Could you check a few things on this model? Use its own coordinates, in mm. A direction names the side the tool comes from. Give positions to 0.01 mm unless a question says otherwise; leave off trailing zeros. Loops run counter-clockwise (first coordinate to the right, second up) from the corner with the lowest first, then second, coordinate; pieces in that order, holes last. Notation, with made-up numbers: M -31,-23.5 L -16,-23.5 A15 ccw -16,-9.5 Z; hole C 43,11 d8. An arc over 180 degrees is marked long. Answer in a Markdown table with one row per item. Add a question column.
```python
from build123d import *

# Parameters (mm, degrees)
ESQUISSE1_W                  = 60
ESQUISSE1_H                  = 60
BOSS_EXTRU_1_DEPTH           = 3
ESQUISSE2_W                  = 40
ESQUISSE2_H                  = 5.064093089
BOSS_EXTRU_2_DEPTH           = 60
ESQUISSE3_R                  = 2.1
ESQUISSE3_W                  = 21
ESQUISSE3_H                  = 42.4
ENL_V_MAT_EXTRU_1_DEPTH      = 61
ESQUISSE4_W                  = 31.43634342
ESQUISSE4_H                  = 7.471813822
BOSS_EXTRU_3_DEPTH           = 49
ENL_V_MAT_EXTRU_2_DEPTH      = 49
ENL_V_MAT_EXTRU_2_DEPTH_BACK = 49
ESQUISSE5_R                  = 2.1
ENL_V_MAT_EXTRU_3_DEPTH      = 5
ENL_V_MAT_EXTRU_3_DEPTH_BACK = 12
ENL_V_MAT_EXTRU_7_DEPTH      = 5.686588472
BOSS_EXTRU_4_DEPTH           = 5
ESQUISSE13_R                 = 1.5
ENL_V_MAT_EXTRU_8_DEPTH      = 5
ENL_V_MAT_EXTRU_9_DEPTH      = 10
CHANFREIN1_SIZE              = 3
CHANFREIN2_SIZE              = 3
ESQUISSE15_R                 = 40.585379392
BOSS_EXTRU_5_DEPTH           = 3
ESQUISSE16_R                 = 4
BOSS_EXTRU_6_DEPTH           = 5.5
ESQUISSE17_R                 = 34
ESQUISSE17_R_2               = 31
BOSS_EXTRU_7_DEPTH           = 1.5


with BuildPart() as part:
    # Esquisse1 → Boss.-Extru.1 (new body)
    with BuildSketch(Plane(origin=(0, 0, 0), x_dir=(1, 0, 0), z_dir=(0, 1, 0))):
        Rectangle(ESQUISSE1_W, ESQUISSE1_H)
    extrude(amount=BOSS_EXTRU_1_DEPTH)

    # Esquisse2 → Boss.-Extru.2 (add)
    with BuildSketch(Plane(origin=(0, 3, 0), x_dir=(1, 0, 0), z_dir=(0, 1, 0))):
        with Locations((0, -27.467953456)):
            Rectangle(ESQUISSE2_W, ESQUISSE2_H)
        with Locations((0, 27.467953456)):
            Rectangle(ESQUISSE2_W, ESQUISSE2_H)
    extrude(amount=BOSS_EXTRU_2_DEPTH)

    # Esquisse3 → Enlèv. mat.-Extru.1 (cut)
    with BuildSketch(Plane.XY.offset(30)):
        with Locations((-5, 57.819250322)):
            Circle(ESQUISSE3_R)
        with Locations((5, 57.819250322)):
            Circle(ESQUISSE3_R)
        with Locations((-5, 7.419250322)):
            Circle(ESQUISSE3_R)
        with Locations((5, 7.419250322)):
            Circle(ESQUISSE3_R)
        with Locations((0, 32.619250322)):
            Rectangle(ESQUISSE3_W, ESQUISSE3_H)
    extrude(amount=-ENL_V_MAT_EXTRU_1_DEPTH, mode=Mode.SUBTRACT)

    # Esquisse4 → Boss.-Extru.3 (add)
    with BuildSketch(Plane(origin=(0, 3, 0), x_dir=(1, 0, 0), z_dir=(0, 1, 0))):
        with Locations((0, 8.9)):
            Rectangle(ESQUISSE4_W, ESQUISSE4_H)
    extrude(amount=BOSS_EXTRU_3_DEPTH)

    # Esquisse5 → Enlèv. mat.-Extru.2 (cut, two sides: drawn at the far end of the back side and taken through both)
    with BuildSketch(Plane.XY.offset(-5.164093089).offset(-ENL_V_MAT_EXTRU_2_DEPTH_BACK)):
        with Locations(Location((0, 41.884866589, 0), (0, 0, 180))):
            Circle(ESQUISSE5_R)
    extrude(amount=ENL_V_MAT_EXTRU_2_DEPTH + ENL_V_MAT_EXTRU_2_DEPTH_BACK, mode=Mode.SUBTRACT)

    # Esquisse6 → Enlèv. mat.-Extru.3 (cut, two sides: drawn at the far end of the back side and taken through both)
    with BuildSketch(Plane.XY.offset(-5.164093089).offset(-ENL_V_MAT_EXTRU_3_DEPTH_BACK)):
        Polygon((3.765814794, 52), (-3.765814794, 52), (-8.396406616, 48.113602092), (-13.009515703, 41.697186725), (-16.070942643, 28.570794505), (-19.383993714, 28.570794505), (-19.383993714, 55.569676943), (19.383993714, 55.569676943), (19.383993714, 28.570794505), (16.070942643, 28.570794505), (13.009515703, 41.697186725), (8.396406616, 48.113602092), align=None)
    extrude(amount=ENL_V_MAT_EXTRU_3_DEPTH + ENL_V_MAT_EXTRU_3_DEPTH_BACK, mode=Mode.SUBTRACT)

    # Esquisse11 → Enlèv. mat.-Extru.7 (cut)
    with BuildSketch(Plane.XY.offset(30)):
        Polygon((-3.554651837, 53.819250322), (0, 57.156758738), (3.554651837, 53.819250322), align=None)
        Polygon((3.554651837, 11.419250322), (0.008232601, 8.05699671), (-3.554651837, 11.419250322), align=None)
    enl_v_mat_extru_7 = extrude(amount=-ENL_V_MAT_EXTRU_7_DEPTH, mode=Mode.SUBTRACT)

    # Symétrie1: Enlèv. mat.-Extru.7 across plane
    add(enl_v_mat_extru_7.mirror(Plane.XY), mode=Mode.SUBTRACT)

    # Esquisse12 → Boss.-Extru.4 (add)
    with BuildSketch(Plane(origin=(0, 0, -30), x_dir=(-1, 0, 0), z_dir=(0, 0, -1))):
        Polygon((-16.041577075, 53.722563772), (-27.510987985, 61.809968901), (-27.510987985, 29.990434482), (-16.041577075, 21.903029354), align=None)
    extrude(amount=-BOSS_EXTRU_4_DEPTH)

    # Esquisse13 → Enlèv. mat.-Extru.8 (cut)
    with BuildSketch(Plane(origin=(0, 0, -30), x_dir=(-1, 0, 0), z_dir=(0, 0, -1))):
        with Locations((-23.733778696, 54.232255727)):
            Circle(ESQUISSE13_R)
    extrude(amount=-ENL_V_MAT_EXTRU_8_DEPTH, mode=Mode.SUBTRACT)

    # Esquisse14 → Enlèv. mat.-Extru.9 (cut)
    with BuildSketch(Plane(origin=(0, 0, -30), x_dir=(-1, 0, 0), z_dir=(0, 0, -1))):
        with BuildLine():
            Line((-21.71817898, 57.725295885), (-22.313097289, 61.571545457))
            Line((-22.313097289, 61.571545457), (-29.123823422, 63.566297114))
            Line((-29.123823422, 63.566297114), (-31.434035617, 54.282245365))
            Line((-31.434035617, 54.282245365), (-31.802093045, 39.80867485))
            Line((-31.802093045, 39.80867485), (-27.510987985, 39.80867485))
            add(Edge.make_bspline(
                [(-27.510987985, 39.80867485), (-27.476511879, 42.426218442), (-27.330002572, 45.177230576), (-27.18875986, 50.317216066), (-27.834123365, 55.293883989), (-23.939343069, 59.432145797), (-21.71817898, 57.725295885)],
                knots=[0, 0, 0, 0, 0.330124206, 0.401515798, 0.713915923, 1, 1, 1, 1], degree=3))
        make_face()
    extrude(amount=-ENL_V_MAT_EXTRU_9_DEPTH, mode=Mode.SUBTRACT)

    # Chanfrein1
    chanfrein1_edges = [part.edges().sort_by_distance(p)[0] for p in [
        (-20, 63, 27.467953456),
        (20, 63, 27.467953456),
        (20, 63, -27.467953456),
        (-20, 63, -27.467953456),
    ]]
    chamfer(chanfrein1_edges, length=CHANFREIN1_SIZE)

    # Chanfrein2
    chanfrein2_edges = [part.edges().sort_by_distance(p)[0] for p in [
        (15.71817171, 3, -8.9),
        (0, 3, -12.635906911),
        (-15.71817171, 3, -8.9),
        (0, 3, -5.164093089),
    ]]
    chamfer(chanfrein2_edges, length=CHANFREIN2_SIZE)

    # Esquisse15 → Boss.-Extru.5 (add)
    with BuildSketch(Plane.XZ):
        Circle(ESQUISSE15_R)
    extrude(amount=-BOSS_EXTRU_5_DEPTH)

    # Esquisse16 → Boss.-Extru.6 (add)
    with BuildSketch(Plane.XZ):
        with Locations(Location((0, 0, 0), (0, 0, 90))):
            Circle(ESQUISSE16_R)
        with BuildLine():
            Line((1.5, -2), (-1.5, -2))
            add(Edge.make_bspline(
                [(-1.5, 2), (-1.958697555, 1.657983746), (-2.533324792, 0.788068376), (-2.517224478, -0.822180507), (-1.942930835, -1.670082257), (-1.5, -2)],
                knots=[0, 0, 0, 0, 0.368917338, 0.642208585, 1, 1, 1, 1], degree=3))
            Line((-1.5, 2), (1.5, 2))
            add(Edge.make_bspline(
                [(1.5, 2), (1.95810566, 1.657096874), (2.561237256, 0.750226685), (2.498088101, -0.878428585), (1.905080516, -1.696028501), (1.5, -2)],
                knots=[0, 0, 0, 0, 0.369168068, 0.672222531, 1, 1, 1, 1], degree=3))
        make_face(mode=Mode.SUBTRACT)
    extrude(amount=BOSS_EXTRU_6_DEPTH)

    # Esquisse17 → Boss.-Extru.7 (add)
    with BuildSketch(Plane.XZ):
        with Locations(Location((0, 0, 0), (0, 0, 90))):
            Circle(ESQUISSE17_R)
        with Locations(Location((0, 0, 0), (0, 0, 270))):
            Circle(ESQUISSE17_R_2, mode=Mode.SUBTRACT)
    extrude(amount=BOSS_EXTRU_7_DEPTH)


solid = part.part
```
Item 1: Suppose I cut it at B-B (x = -22). List the corners of the cut face in (y, z) for me, then the cut area to 3 significant figures.
Item 2: If we mould it in two halves opening along Z, with no side actions, what happens to faces 1 (the face through (4.54, 5.37, -27.43)), 2 (the face through (-0.262, 4.521, -14.115)), 3 (the face through (0, -3, -2))? For each: +Z half, -Z half, draft (parallel to the pull), parting line (faces both ways), or undercut.
Item 3: For P1, Ø4, axis at x = -6.5, z = -28.5, coming from the -Y side; P2, Ø24, axis at x = 10, y = 38.5, coming from the -Z side; P3, Ø1, axis at x = -18, y = 20.5, coming from the +Z side, each with a flat end and sliding along its axis, tell me the tip position at first contact or that it passes through.
Item 4: Suppose I cut it at A-A (z = -8.5). List the corners of the cut face in (x, y) for me.
Item 5: For faces 4 (the face through (10.5, 32, 28)), 5 (the face through (10.735, 44.86, -8.952)), 6 (the face through (-1.802, 55.465, -27.503)), 7 (the face through (-30, 1, 29)), which set-ups out of +Z, -Z, +X, -X, +Y, -Y let a thin tool reach every point of the face, with its end or its side?
Item 6: I need wall thicknesses on L1, parallel to Y at x = 5, z = -28; L2, parallel to Y at x = 0, z = -10; L3, parallel to Z at x = -12, y = 51. Which ranges of each line are inside material? Lowest first, please.
Item 7: Suppose I cut it at C-C (z = 20). List the corners of the cut face in (x, y) for me.
Item 8: Suppose I cut it at D-D (z = -36). List the corners of the cut face in (x, y) for me.
Values found:
| question | item | result |
|---|---|---|
| 1 | outline | M -1.5,-25.92 L 0,-25.92 L 0,-34.11 L 3,-34.11 L 3,34.11 L 0,34.11 L 0,25.92 L -1.5,25.92 L -1.5,21.84 L 0,21.84 L 0,-21.84 L -1.5,-21.84 Z |
| 1 | area | 217 mm² |
| 2 | face 1 | draft |
| 2 | face 2 | undercut |
| 2 | face 3 | undercut |
| 3 | P1 | y = -1.5 |
| 3 | P2 | z = -30 |
| 3 | P3 | z = 30 |
| 4 | outline | M -39.69,0 L -32.92,0 L -32.92,-1.5 L -29.81,-1.5 L -29.81,0 L 29.81,0 L 29.81,-1.5 L 32.92,-1.5 L 32.92,0 L 39.69,0 L 39.69,3 L 18.72,3 L 15.72,6 L 15.72,30.08 L 13.01,41.7 L 8.4,48.11 L 3.77,52 L -3.77,52 L -8.4,48.11 L -13.01,41.7 L -15.72,30.08 L -15.72,6 L -18.72,3 L -39.69,3 Z; hole C 0,41.88 d4.2 |
| 5 | face 4 | +Z |
| 5 | face 5 | +X, +Y |
| 5 | face 6 | +Z, -Z |
| 5 | face 7 | +Z, -X, +Y, -Y |
| 6 | L1 | 0 to 5.32, 9.52 to 11.42, 53.82 to 55.72, 59.92 to 63 |
| 6 | L2 | 0 to 39.78, 43.98 to 52 |
| 6 | L3 | -30 to -24.94, 24.94 to 30 |
| 7 | outline | M -35.32,0 L -27.5,0 L -27.5,-1.5 L -23.69,-1.5 L -23.69,0 L 23.69,0 L 23.69,-1.5 L 27.5,-1.5 L 27.5,0 L 35.32,0 L 35.32,3 L -35.32,3 Z |
| 8 | outline | M -18.74,0 L 18.74,0 L 18.74,3 L -18.74,3 Z |
